For this review, take the finished solid that the model builds, in its own axes (mm). A direction names the side the tool comes from. Coordinates: 2 decimals unless noted, no trailing zeros. Order: outer loops, then holes, each group sorted by start corner. A loop starts at its lowest first (then second) coordinate and runs counter-clockwise, first axis right, second up.
from build123d import *

# Parameters (mm, degrees)
BOSS_EXTRUDE1_DEPTH  = 225
FILLET1_R            = 6.35
SKETCH2_R            = 15
CUT_EXTRUDE1_DEPTH   = 75
CUT_EXTRUDE2_DEPTH   = 10
M6_CLEARANCE_HOLE1_D = 6.4


with BuildPart() as part:
    # Sketch1 → Boss-Extrude1 (new body)
    with BuildSketch(Plane(origin=(0, 0, 0), x_dir=(0, 0, -1), z_dir=(1, 0, 0))):
        with BuildLine():
            Line((0, 0), (0, 101.6))
            Line((0, 101.6), (6.35, 101.6))
            Line((6.35, 101.6), (6.35, 15.875))
            ThreePointArc((6.35, 15.875), (9.139807909, 9.139807909), (15.875, 6.35))
            Line((15.875, 6.35), (40, 6.35))
            Line((40, 6.35), (40, 0))
            Line((40, 0), (0, 0))
        make_face()
    extrude(amount=BOSS_EXTRUDE1_DEPTH)

    # Fillet1
    fillet1_edges = [part.edges().sort_by_distance(p)[0] for p in [
        (112.5, 0, 0),
    ]]
    fillet(fillet1_edges, radius=FILLET1_R)

    # Sketch2 → Cut-Extrude1 (cut)
    with BuildSketch(Plane(origin=(0, 0, 0), x_dir=(-1, 0, 0), z_dir=(0, 0, -1))):
        with Locations((-37.5, 70)):
            Circle(SKETCH2_R)
        with Locations((-187.5, 70)):
            Circle(SKETCH2_R)
    extrude(amount=CUT_EXTRUDE1_DEPTH, mode=Mode.SUBTRACT)

    # Sketch5 → Cut-Extrude2 (cut)
    with BuildSketch(Plane(origin=(0, 0, -6.35), x_dir=(-1, 0, 0), z_dir=(0, 0, -1))):
        with BuildLine():
            Line((-107.5, 44.875), (-107.5, 26.875))
            ThreePointArc((-107.5, 26.875), (-112.5, 21.875), (-117.5, 26.875))
            Line((-117.5, 26.875), (-117.5, 44.875))
            ThreePointArc((-117.5, 44.875), (-112.5, 49.875), (-107.5, 44.875))
        make_face()
    extrude(amount=-CUT_EXTRUDE2_DEPTH, mode=Mode.SUBTRACT)

    # M6 Clearance Hole1 (through all)
    with Locations(Plane(origin=(20, 0, -25), x_dir=(0, 0, -1), z_dir=(0, -1, 0))):
        with Locations((0, 0), (0, 50), (0, 135), (0, 185)):
            Hole(M6_CLEARANCE_HOLE1_D / 2)


solid = part.part
1. Take a section at D-D, the plane x = 122. Give the boundary of the cut face in (y, z) (3 decimals).
Answer below:
outline: (0, -40) - (6.35, -40) - (6.35, -15.875) arc R9.525 cw to (15.875, -6.35) - (101.6, -6.35) - (101.6, 0) - (6.35, 0) arc R6.35 ccw to (0, -6.35) - close
2. The part is to be moulded in two halves that separate along Y. For faces 4 (the face through (117.5, 36, -3)), 5 (the face through (114.08, 1.91, -1.81)), 6 (the face through (40.752, 55.357, -3.131)), 7 (the face through (20.1, 3.2, -28.2)), say which applies: +Y half, -Y half, draft (parallel to the pull), parting line (faces both ways), or undercut.
Answer below:
face 4: undercut
face 5: -Y half
face 6: undercut
face 7: draft
3. Take a section at C-C, the plane z = -24.5. Give the boundary of the cut face in (x, y), plus the area to 3 significant figures.
Answer below:
outline: (0, 0) - (16.84, 0) - (16.84, 6.35) - (0, 6.35) - close; (23.16, 0) - (66.84, 0) - (66.84, 6.35) - (23.16, 6.35) - close; (73.16, 0) - (151.84, 0) - (151.84, 6.35) - (73.16, 6.35) - close; (158.16, 0) - (201.84, 0) - (201.84, 6.35) - (158.16, 6.35) - close; (208.16, 0) - (225, 0) - (225, 6.35) - (208.16, 6.35) - close
area: 1,270 mm2
4. Machinability: for faces 1 (the face through (111, 6.35, -28)), 2 (the face through (225, 36, -5)), 3 (the face through (107.5, 36, -3)), which of the approach directions +Z, -Z, +X, -X, +Y, -Y give a long, thin tool a straight path to every point of the face, cutting with its end or side? Answer none if there is none.
Answer below:
face 1: -Z, +X, -X, +Y
face 2: +Z, -Z, +X, +Y, -Y
face 3: +Z, -Z
5. To check wall thickness, follow L1, parallel to X at y = 4, z = -25; L2, parallel to X at y = 70, z = -4; L3, parallel to X at y = 75, z = -5. State the ranges of each line that lie inside material, in increasing order.
Answer below:
L1: x = 0 to 16.8, 23.2 to 66.8, 73.2 to 151.8, 158.2 to 201.8, 208.2 to 225
L2: x = 0 to 22.5, 52.5 to 172.5, 202.5 to 225
L3: x = 0 to 23.36, 51.64 to 173.36, 201.64 to 225
6. Clearance check with flat-ended pins moving along their axes: pin 1 Ø5 at (x, z) = (45.5, -20.5) entering from +Y; pin 2 Ø6 at (x, z) = (70, -25) entering from -Y; pin 3 Ø1.9 at (y, z) = (33.5, -3.5) entering from -X; pin 4 Ø5 at (x, y) = (78.5, 84) entering from -Z. State where each tip first meets the part, or that it passes through.
Answer below:
pin 1: stops at y = 6.35
pin 2: passes through
pin 3: stops at x = 0
pin 4: stops at z = -6.35
7. Take a section at A-A, the plane x = 187.5. Give the boundary of the cut face in (y, z) (3 decimals).
Answer below:
outline: (0, -40) - (6.35, -40) - (6.35, -15.875) arc R9.525 cw to (15.875, -6.35) - (55, -6.35) - (55, 0) - (6.35, 0) arc R6.35 ccw to (0, -6.35) - close; (85, -6.35) - (101.6, -6.35) - (101.6, 0) - (85, 0) - close
8. Take a section at B-B, the plane y = 60. Give the boundary of the cut face in (x, z), plus the area to 3 significant figures.
Answer below:
outline: (0, -6.35) - (26.32, -6.35) - (26.32, 0) - (0, 0) - close; (48.68, -6.35) - (176.32, -6.35) - (176.32, 0) - (48.68, 0) - close; (198.68, -6.35) - (225, -6.35) - (225, 0) - (198.68, 0) - close
area: 1,140 mm2
